Check sheet for the modelled part. Datum: model origin and axes. Units: mm. Face numbers are marked on the shaded views. A direction names the side the tool comes from. Give positions to 0.01 mm unless a question says otherwise; leave off trailing zeros. Order: outer loops, then holes, each group sorted by start corner. A loop starts at its lowest first (then second) coordinate and runs counter-clockwise, first axis right, second up. Notation, with made-up numbers: (38, 87) - (81, 87) arc R21 ccw to (81, 118) - close; hole circle Ø7 at (-30.75, 62). An arc over 180 degrees is marked (long way). Answer in a Markdown table with one row per item.
from build123d import *

# Parameters (mm, degrees)
F1_DEPTH = 10


with BuildPart() as f1:
    # F0 (on Top) → F1 (new body)
    with BuildSketch(Plane.XY):
        with BuildLine():
            Line((8, -20), (8, 20))
            Line((8, 20), (4, 20))
            ThreePointArc((4, 20), (0, 16), (-4, 20))
            Line((-4, 20), (-8, 20))
            Line((-8, 20), (-8, -20))
            Line((-8, -20), (-13, -20))
            Line((-13, -20), (-13, -30))
            Line((-13, -30), (13, -30))
            Line((13, -30), (13, -20))
            Line((13, -20), (8, -20))
        make_face()
    extrude(amount=F1_DEPTH)


solid = f1.part
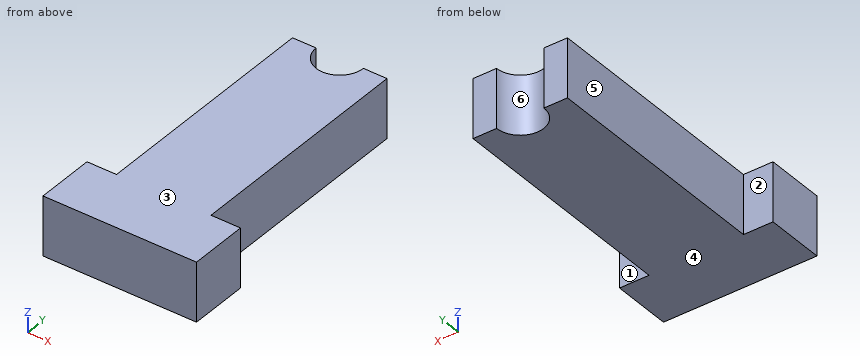
(1) Thickness scan on L1, parallel to Y at x = 8.5, z = 7; L2, parallel to X at y = -7.5, z = 3.5; L3, parallel to Y at x = 1.5, z = 6.25. Record the ranges inside material, lowest first.
Geometry says:
| item | result |
|---|---|
| L1 | -30 to -20 |
| L2 | -8 to 8 |
| L3 | -30 to 16.29 |
(2) Mould release check, pull along X, two halves, no side actions. Record for the marked faces 4, 5 and 6: pulls with the +X half, pulls with the -X half, needs draft (parallel to the pull), parting line crosses it, or undercut.
Geometry says:
| item | result |
|---|---|
| face 4 | needs draft |
| face 5 | pulls with the -X half |
| face 6 | undercut |
(3) Cross-section at B-B, the plane x = 0. Record the cut outline in (y, z), then the cut area to 3 significant figures.
Geometry says:
| item | result |
|---|---|
| outline | (-30, 0) - (16, 0) - (16, 10) - (-30, 10) - close |
| area | 460 mm² |
(4) Gauge pin test, flat ends, axial feed: P1, Ø5, axis at y = -2.5, z = 4.5, coming from the +X side; P2, Ø3, axis at x = 10, y = 3.5, coming from the -Z side; P3, Ø1.5, axis at x = -10.5, z = 6, coming from the +Y side; P4, Ø1, axis at y = 4.5, z = 2, coming from the -X side. Record the tip position at first contact, or that the pin passes through.
Geometry says:
| item | result |
|---|---|
| P1 | x = 8 |
| P2 | through |
| P3 | y = -20 |
| P4 | x = -8 |
(5) Access from +Z, -Z, +X, -X, +Y, -Y to the whole of each face (thin tool, end or side, straight path). Record for the marked faces 1, 2 and 3.
Geometry says:
| item | result |
|---|---|
| face 1 | +Z, -Z, +X, +Y |
| face 2 | +Z, -Z, -X, +Y |
| face 3 | +Z, +X, -X, +Y, -Y |
(6) Cross-section at A-A, the plane z = 1. Record the cut outline in (x, y), then the cut area to 3 significant figures.
Geometry says:
| item | result |
|---|---|
| outline | (-13, -30) - (13, -30) - (13, -20) - (8, -20) - (8, 20) - (4, 20) arc R4 cw to (-4, 20) - (-8, 20) - (-8, -20) - (-13, -20) - close |
| area | 875 mm² |
(7) Cross-section at C-C, the plane y = 13.5. Record the cut outline in (x, z), then the cut area to 3 significant figures.
Geometry says:
| item | result |
|---|---|
| outline | (-8, 0) - (8, 0) - (8, 10) - (-8, 10) - close |
| area | 160 mm² |
